Geometry check sheet. Reference: the model listing, model coordinates, mm. A direction names the side the tool comes from. Give positions to 0.01 mm unless a question says otherwise; leave off trailing zeros. Write each loop counter-clockwise with the first axis right and the second up, starting at its lowest first coordinate (ties: lowest second). Pieces come first, ordered by that corner, then holes. Notation, with made-up numbers: (51, -2.5) - (107, -2.5) arc R16 cw to (107, 15.5) - close; hole circle Ø7 at (21.25, -9.75). An arc over 180 degrees is marked (long way). Write item = value, one per line. Start each with the question number.
(1) Access from +Z, -Z, +X, -X, +Y, -Y to the whole of each face (thin tool, end or side, straight path). Record for faces 4 (the flat face through (32, 10, -4)), 5 (the flat face through (32, 10, 0)), 6 (the cylindrical face through (1.14, 18.9, -2.03)).
(2) Section check C-C, the plane y = -3. Enter the section's corners in (x, z).
(3) Thickness scan on L1, parallel to X at y = 2.25, z = 12.5; L2, parallel to Z at x = 10, y = 1.85; L3, parallel to X at y = 1.5, z = 11.75. Record the ranges inside material, lowest first.
(4) Section check B-B, the plane z = 12.5. Enter the section's corners in (x, y), plus the area to 3 significant figures.
(5) Depth check by flat-ended pin: pin 1 Ø22 at (x, y) = (38.5, 11.5) entering from -Z; pin 2 Ø10 at (x, y) = (27, -4) entering from -Z; pin 3 Ø8 at (x, z) = (24.5, 9.5) entering from -Y. Enter the tip coordinate at first touch or a pass-through.
(6) Draft check along Y on faces 1 (the cylindrical face through (63.86, 18.9, -1.97)), 2 (the cylindrical face through (14.55, -15.76, -3.4)), 3 (the cylindrical face through (56.335, 1.972, 12.921)). Enter one of: pulls with the +Y half, pulls with the -Y half, needs draft (parallel to the pull), parting line crosses it, or undercut.
Autodesk Fusion 360 part; units mm, degrees
sketch "草图6" plane through (0, 0, 0) normal (0, 1, 0) x (1, 0, 0)
  line L0 (0, 0) -> (65, 0)
  line L1 (65, 0) -> (65, -19.5)
  line L2 (65, -19.5) -> (0, -19.5)
  line L3 (0, -19.5) -> (0, 0)
  line L4 (0, 0) -> (0, 4)
  line L5 (0, 4) -> (65, 4)
  line L6 (65, 4) -> (65, 0)
  circle A0 centre (10, -12.5) radius 1.4
  circle A1 centre (55, -12.5) radius 1.4
  line L7 (32.5, -19.5) -> (32.5, 4) construction
  dimension "d31" = 65
  dimension "d32" = 19.5
  dimension "d33" = 4
  dimension "d34" = 7
  dimension "d35" = 2.8
  dimension "d36" = 45
extrude "拉伸5" add sketch "草图6" along normal blind 4 contours L0 L1 L2 L3 makes body 1
extrude "拉伸6" add sketch "草图6" along normal blind 20.105 contours L0 L4 L5 L6 bodies 1
sketch "草图7" plane through (0, 0, 0) normal (0, 0, 1) x (1, 0, 0)
  line L0 (0, 4) -> (65, 4)
  line L1 (65, 4) -> (65, 20.105)
  line L2 (65, 20.105) -> (0, 20.105)
  line L3 (0, 20.105) -> (0, 4)
  circle A0 centre (32.5, 14.15) radius 3.325
  line L4 (32.5, 4) -> (32.5, 20.105) construction
  circle A1 centre (32.5, 14.15) radius 3.825
  dimension "d41" = 10.15
  dimension "d42" = 6.65
  dimension "d43" = 7.65
extrude "拉伸7" cut sketch "草图7" against normal blind 4 contours A0 bodies 1
extrude "拉伸8" cut sketch "草图7" against normal blind 0.5 contours A1 bodies 1
chamfer "倒角1" distance 0.5 angle 45 1 edges at (28.9338, 15.5332, -0.5) on bodies 1
fillet "圆角1" radius 4 1 edges at (0, 2, 19.5) on bodies 1
fillet "圆角2" radius 4 1 edges at (65, 2, 19.5) on bodies 1
fillet "圆角3" radius 1 1 edges at (32.5, 4, 0) on bodies 1
fillet "圆角4" radius 4 1 edges at (32.5, 0, -4) on bodies 1
fillet "圆角5" radius 4 1 edges at (0, 20.105, -2) on bodies 1
fillet "圆角6" radius 4 1 edges at (65, 20.105, -2) on bodies 1
delete_face "删除面1" 1 faces at (21.6667, 3.8097, -3.9955) on bodies 1
ref_plane "工作平面1" through (32.5, 0, -4) normal (0, -0.0872, 0.9962) x (1, 0, 0)
sketch "草图8" plane through (0, 0.3473, -3.9696) normal (0, -0.0872, 0.9962) x (1, 0, 0)
  line L0 (0, -0.3486) -> (65, -0.3486)
  line L1 (0, -0.3486) -> (0, -30.3486)
  line L2 (0, -30.3486) -> (65, -30.3486)
  line L3 (65, -30.3486) -> (65, -0.3486)
  line L4 (0, -15.3486) -> (65, -15.3486) construction
  circle A0 centre (12.5, -15.3486) radius 2.15
  line L5 (32.5, -0.3486) -> (32.5, -30.3486) construction
  circle A1 centre (52.5, -15.3486) radius 2.15
  point P0 (0, -0.3486)
  point P1 (65, -0.3486)
  dimension "d62" = 30
  dimension "d64" = 4.3
  dimension "d65" = 40
extrude "拉伸9" add sketch "草图8" along normal blind 4 separate body makes body 2
extrude "拉伸10" add 1 faces at (21.6667, -0.2324, -1.3435) along direction (0, 0.996195, 0.087156) blind 0.877 on bodies 2 bodies 1 2
fillet "圆角7" radius 4 2 edges at (65, -30.0602, -4.6223) (0, -30.0602, -4.6223) on bodies 1
fillet "圆角8" radius 4 1 edges at (32.5, 0, 0.0153) on bodies 1
delete_face "删除面2" 1 faces at (43.3333, -3.2596, -0.2503) on bodies 1
delete_face "删除面3" 1 faces at (21.6667, 4.4199, 0.1854) on bodies 1
extrude "拉伸3" [suppressed]
sketch "草图4" plane through (0, 0, 0) normal (0, 1, 0) x (1, 0, 0)
  line L0 (0, 0) -> (65, 0)
  line L1 (65, 0) -> (65, -25.17)
  line L2 (65, -25.17) -> (0, -25.17)
  line L3 (0, -25.17) -> (0, 0)
  line L4 (0, -7) -> (65, -7) construction
  circle A0 centre (10, -7) radius 1.25
  line L5 (32.5, 0) -> (32.5, -25.17) construction
  circle A1 centre (55, -7) radius 1.25
  line L6 (0, -21.17) -> (65, -21.17)
  dimension "d23" = 25.17
  dimension "d24" = 65
  dimension "d25" = 2.5
  dimension "d26" = 45
  dimension "d27" = 7
  dimension "d28" = 4
extrude "拉伸4" [suppressed]
sketch "草图5" plane through (0, 0, 25.17) normal (0, 0, 1) x (1, 0, 0)
  line L0 (0, 0) -> (65, 0)
  line L1 (65, 0) -> (65, 4)
  line L2 (65, 4) -> (0, 4)
  line L3 (0, 4) -> (0, 0)
equation "d23 = 14 mm + 7.17 mm + 4 mm"
equation "d39 = 16.105 mm + 4 mm"
Model answer:
q1.face_4 = -Z, +X, -X, +Y
q1.face_5 = +Z, +X, -X, +Y
q1.face_6 = +Z, -Z, -X, +Y
q2.outline = (0, -4.26) - (65, -4.26) - (65, -0.25) - (0, -0.25) - close
q3.L1 = 0 to 8.6, 11.4 to 53.6, 56.4 to 65
q3.L2 = -4 to 11.1, 13.9 to 19.5
q3.L3 = 0 to 8.82, 11.18 to 53.82, 56.18 to 65
q4.outline = (0, 0) - (8.6, 0) - (8.6, 4) - (0, 4) - close; (11.4, 0) - (53.6, 0) - (53.6, 4) - (11.4, 4) - close; (56.4, 0) - (65, 0) - (65, 4) - (56.4, 4) - close
q4.area = 238 mm²
q5.pin_1 = -4
q5.pin_2 = -4.79
q5.pin_3 = 0
q6.face_1 = pulls with the +Y half
q6.face_2 = undercut
q6.face_3 = needs draft
